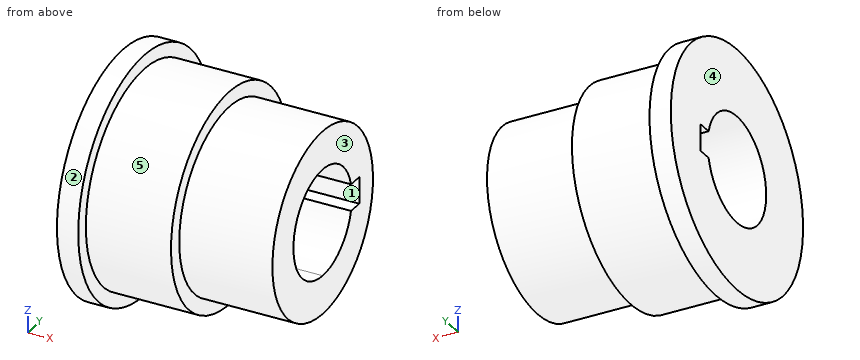
```python
from build123d import *

# Parameters (mm, degrees)
SKETCH1_R           = 10.9140625
BOSS_EXTRUDE1_DEPTH = 23.8125
SKETCH2_R           = 12.7
SKETCH2_R_2         = 10.9140625
BOSS_EXTRUDE2_DEPTH = 12.7
SKETCH5_R           = 14.351
SKETCH5_R_2         = 12.7
BOSS_EXTRUDE3_DEPTH = 2.54


with BuildPart() as part:
    # Sketch1 → Boss-Extrude1 (new body)
    with BuildSketch(Plane(origin=(0, 0, 0), x_dir=(0, 0, -1), z_dir=(1, 0, 0))):
        Circle(SKETCH1_R)
        with BuildLine():
            Line((-1.5875, 6.148361062), (-1.5875, 7.9375))
            Line((-1.5875, 7.9375), (1.5875, 7.9375))
            Line((1.5875, 7.9375), (1.5875, 6.148361062))
            ThreePointArc((1.5875, 6.148361062), (5.020115786, 3.888564967), (6.35, 0))
            ThreePointArc((6.35, 0), (-3.888564967, -5.020115786), (-1.5875, 6.148361062))
        make_face(mode=Mode.SUBTRACT)
    extrude(amount=BOSS_EXTRUDE1_DEPTH)

    # Sketch2 → Boss-Extrude2 (add)
    with BuildSketch(Plane.ZY):
        Circle(SKETCH2_R)
        Circle(SKETCH2_R_2, mode=Mode.SUBTRACT)
    extrude(amount=-BOSS_EXTRUDE2_DEPTH)

    # Sketch5 → Boss-Extrude3 (add)
    with BuildSketch(Plane.ZY):
        Circle(SKETCH5_R)
        Circle(SKETCH5_R_2, mode=Mode.SUBTRACT)
    extrude(amount=-BOSS_EXTRUDE3_DEPTH)


solid = part.part
```
Model file for the job. Use its own axes, mm. Face numbers are marked on the shaded views. A direction names the side the tool comes from. Coordinates: 2 decimals unless noted, no trailing zeros. Order: outer loops, then holes, each group sorted by start corner. A loop starts at its lowest first (then second) coordinate and runs counter-clockwise, first axis right, second up. Notation, with made-up numbers: (-6.5, 56.25) - (32.5, 56.25) arc R37 cw to (32.5, 92.25) - close; hole circle Ø9 at (-8.5, -16). An arc over 180 degrees is marked (long way). Return JSON: item names as keys, results as strings. Group by question number.
1) Mould opens along Y. For the marked faces 1, 2 and 3 say: released by +Y, released by -Y, zero draft, split by the parting line, or undercut.
2) Saw through at D-D, the plane y = -10.25. Write the cut outline in (x, z).
3) Saw through at A-A, the plane z = 0. Write the cut outline in (x, y), plus the area to 3 significant figures.
4) Saw through at C-C, the plane y = 4.25. Write the cut outline in (x, z).
5) Flat gauge pins, fed straight in: P1, Ø8, axis at y = -4, z = 0, coming from the -X side; P2, Ø1.5, axis at x = 8.5, y = 2, coming from the +Z side; P3, Ø0.5, axis at x = 8.5, y = 7, coming from the -Z side; P4, Ø6, axis at x = 10, z = 4.5, coming from the +Y side. Where does each tip first touch, or does it go through?
6) Saw through at B-B, the plane x = 14.5. Write the cut outline in (y, z).
7) Tool access for the marked faces 4 and 5: list every direction of +Z, -Z, +X, -X, +Y, -Y with a clear straight run to the whole face (end or side of a thin tool).
8) Probe line 1 (Y direction, x = 7, z = 0); line 2 (X direction, y = -8, z = 8); line 3 (Y direction, x = 13.75, z = 3.5). List the from-to ranges inside material, lowest first. Write a range as from..to.
Values found:
{
 "1": {"face 1": "undercut", "face 2": "split by the parting line", "face 3": "zero draft"},
 "2": {"outline": "(0, -10.04) - (2.54, -10.04) - (2.54, -7.5) - (12.7, -7.5) - (12.7, -3.75) - (23.81, -3.75) - (23.81, 3.75) - (12.7, 3.75) - (12.7, 7.5) - (2.54, 7.5) - (2.54, 10.04) - (0, 10.04) - close"},
 "3": {"outline": "(0, -14.35) - (2.54, -14.35) - (2.54, -12.7) - (12.7, -12.7) - (12.7, -10.91) - (23.81, -10.91) - (23.81, -6.35) - (0, -6.35) - close; (0, 7.94) - (23.81, 7.94) - (23.81, 10.91) - (12.7, 10.91) - (12.7, 12.7) - (2.54, 12.7) - (2.54, 14.35) - (0, 14.35) - close", "area": "233 mm²"},
 "4": {"outline": "(0, -13.71) - (2.54, -13.71) - (2.54, -11.97) - (12.7, -11.97) - (12.7, -10.05) - (23.81, -10.05) - (23.81, -4.72) - (0, -4.72) - close; (0, 4.72) - (23.81, 4.72) - (23.81, 10.05) - (12.7, 10.05) - (12.7, 11.97) - (2.54, 11.97) - (2.54, 13.71) - (0, 13.71) - close"},
 "5": {"P1": "stops at x = 0", "P2": "stops at z = 12.64", "P3": "stops at z = -10.76", "P4": "stops at y = 12.61"},
 "6": {"outline": "circle Ø21.83 at (0, 0); hole (6.15, -1.59) - (7.94, -1.59) - (7.94, 1.59) - (6.15, 1.59) arc R6.35 ccw (long way) to start"},
 "7": {"face 4": "+Z, -Z, -X, +Y, -Y", "face 5": "+X"},
 "8": {"line 1": "y = -12.7..-6.35, 7.94..12.7", "line 2": "x = 0..12.7", "line 3": "y = -10.34..-5.3, 5.3..10.34"}
}
